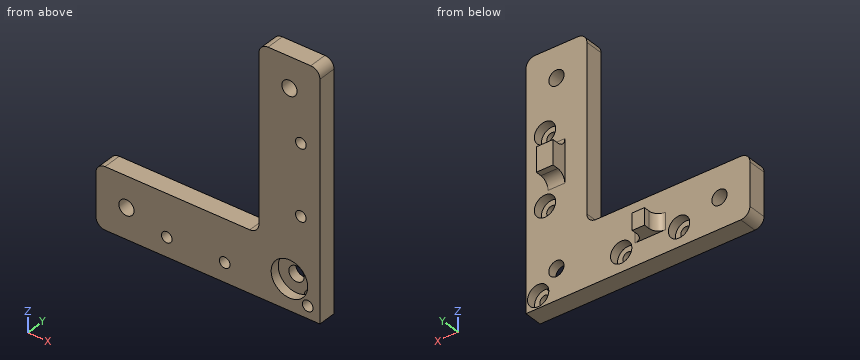
Autodesk Inventor part; units mm, degrees
ref_plane "YZ Plane" through (0, 0, 0) normal (1, 0, 0) x (0, 1, 0)
ref_plane "XZ Plane" through (0, 0, 0) normal (0, 1, 0) x (-1, 0, 0)
ref_plane "XY Plane" through (0, 0, 0) normal (0, 0, 1) x (1, 0, 0)
sketch "Эскиз1" plane through (0, 0, 0) normal (0, 1, 0) x (-1, 0, 0)
  line L0 (0, 0) -> (0, 80)
  line L1 (0, 80) -> (20, 80)
  line L2 (20, 80) -> (20, 20)
  line L3 (20, 20) -> (73.5, 20)
  line L4 (73.5, 20) -> (73.5, 0)
  line L5 (73.5, 0) -> (0, 0)
  dimension "d0" = 80
  dimension "d1" = 20
  dimension "d2" = 60
  dimension "d3" = 53.5
extrude "Выдавливание1" add sketch "Эскиз1" along normal blind 6
fillet "Сопряжение1" radius 3 5 edges at (-73.5, 3, 20) (-73.5, 3, 0) (-20, 3, 80) (0, 3, 80) (-20, 3, 20)
sketch "Эскиз2" plane through (0, 6, 0) normal (0, 1, 0) x (1, 0, 0)
  circle A0 centre (-6.25, -31.25) radius 1.75
  circle A1 centre (-4, -4) radius 1.75
  circle A2 centre (-31.25, -6.25) radius 1.75
  circle A3 centre (-50.25, -6.25) radius 1.75
  circle A4 centre (-6.25, -54.25) radius 1.75
  circle A5 centre (-6.25, -54.25) radius 3.5
  circle A6 centre (-6.25, -31.25) radius 3.5
  circle A7 centre (-4, -4) radius 3.5
  circle A8 centre (-31.25, -6.25) radius 3.5
  circle A9 centre (-50.25, -6.25) radius 3.5
  dimension "d7" = 7
  dimension "d8" = 7
  dimension "d9" = 7
  dimension "d10" = 7
  dimension "d11" = 7
extrude "Выдавливание2" cut sketch "Эскиз2" against normal through all contours A0 | A1 | A2 | A3 | A4
extrude "Выдавливание3" cut sketch "Эскиз2" against normal blind 3 contours A0 | A1 | A2 | A3 | A4 | A5 | A6 | A7 | A8 | A9
sketch "Эскиз3" plane through (0, 6, 0) normal (0, 1, 0) x (1, 0, 0)
  line L0 (-20, -85.5935) -> (0, -85.5935)
  line L1 (-7.25, -46.75) -> (-12.75, -46.75)
  line L2 (-12.75, -46.75) -> (-12.75, -38.75)
  line L3 (-12.75, -38.75) -> (-7.25, -38.75)
  line L4 (-7.25, -38.75) -> (-7.25, -46.75)
  line L5 (-7.25, -46.75) -> (-12.75, -38.75) construction
  line L6 (-12.75, -46.75) -> (-7.25, -38.75) construction
  line L7 (0, 0) -> (13.4319, 0) construction
  line L8 (-42.75, -12.75) -> (-38.75, -12.75)
  line L9 (-38.75, -12.75) -> (-38.75, -7.25)
  line L10 (-38.75, -7.25) -> (-42.75, -7.25)
  line L11 (-42.75, -7.25) -> (-42.75, -12.75)
  point P0 (-10, -42.75)
extrude "Выдавливание4" add sketch "Эскиз3" along normal blind 5
sketch "Эскиз4" plane through (0, 6, 0) normal (0, 1, 0) x (1, 0, 0)
  line L0 (-27.1384, -80) -> (-27.1384, -70)
  line L1 (-80, 9.988) -> (-53.75, 9.988)
  circle A0 centre (-10, -70) radius 2.5
  line L2 (-73.5, -29.8806) -> (-63.5, -29.8806)
  circle A1 centre (-63.5, -10) radius 2.5
  point P0 (0, 0)
  dimension "d26" = 10
  dimension "d27" = 5
  dimension "d28" = 10
  dimension "d29" = 5
extrude "Выдавливание5" cut sketch "Эскиз4" against normal through all
sketch "Эскиз5" plane through (0, 0, 0) normal (0, -1, 0) x (1, 0, 0)
  line L0 (0, 77) -> (0, 0)
  line L1 (0, 0) -> (-10, 0)
  line L2 (-10, 0) -> (-10, 10)
  line L3 (-10, 10) -> (0, 10)
  line L4 (0, 10) -> (0, 0)
  circle A0 centre (-10, 10) radius 2.5
  circle A1 centre (-10, 10) radius 6
  dimension "d32" = 10
  dimension "d33" = 10
  dimension "d34" = 5
  dimension "d35" = 12
extrude "Выдавливание6" cut sketch "Эскиз5" against normal through all contours A0 L2 L3 | L3 L2 A0
extrude "Выдавливание7" cut sketch "Эскиз5" against normal blind 3 contours A1 L2 A0 L3 | L3 A0 L2 A1 | A0 L2 L3 | L3 L2 A0
fillet "Сопряжение2" radius 3 4 edges at (-42.75, 6, 10) (-38.75, 6, 10) (-10, 6, 38.75) (-10, 6, 46.75)
properties part number "perehodnik"
Here's how the part is built. I have some questions about the finished solid (model axes, mm). Give positions to 0.01 mm unless a question says otherwise; leave off trailing zeros. Write each loop counter-clockwise with the first axis right and the second up, starting at its lowest first coordinate (ties: lowest second). Pieces come first, ordered by that corner, then holes. Notation, with made-up numbers: (11.5, -31.75) -> (18.5, -31.75) arc R20 ccw to (18.5, 6.25) -> close; hole circle Ø7 at (48.25, 56.5). An arc over 180 degrees is marked (long way). Write each question's results on one line, items separated by ' | '.
Item 1: Suppose I cut it at C-C on x = -63.5. Write out the boundary of the cut face in (y, z), plus the area to 3 significant figures.
Output:
outline: (0, 0) -> (6, 0) -> (6, 7.5) -> (0, 7.5) -> close; (0, 12.5) -> (6, 12.5) -> (6, 20) -> (0, 20) -> close | area: 90.0 mm^2
Item 2: Suppose I cut it at B-B on y = 4. Give the number of separate pieces and of enclosed holes in the cut face, plus the area to 3 significant figures.
Output:
separate pieces: 1 | enclosed holes: 8 | area: 2,410 mm^2
Item 3: If I drill on L1, parallel to X at y = 4.75, z = 31.25; L2, parallel to Z at x = -10, y = 0.9; L3, parallel to X at y = 2.05, z = 31.25, over which ranges is the centre line in solid material (lowest first)?
Output:
L1: x = -20 to -9.75, -2.75 to 0 | L2: z = 0 to 4, 16 to 67.5, 72.5 to 80 | L3: x = -20 to -8, -4.5 to 0
Item 4: Suppose I cut it at D-D on z = 31.25. Write out the boundary of the cut face in (x, y).
Output:
outline: (-20, 0) -> (-8, 0) -> (-8, 3) -> (-9.75, 3) -> (-9.75, 6) -> (-20, 6) -> close; (-4.5, 0) -> (0, 0) -> (0, 6) -> (-2.75, 6) -> (-2.75, 3) -> (-4.5, 3) -> close
Item 5: Suppose I cut it at A-A on z = 70. Write out the boundary of the cut face in (x, y).
Output:
outline: (-20, 0) -> (-12.5, 0) -> (-12.5, 6) -> (-20, 6) -> close; (-7.5, 0) -> (0, 0) -> (0, 6) -> (-7.5, 6) -> close
Item 6: For pin 1 Ø5.5 at (x, y) = (-43, 8.5) entering from +Z; pin 2 Ø3.5 at (x, z) = (-4, 3.5) entering from +Y; pin 3 Ø3.5 at (x, z) = (-13, 12) entering from -Y; pin 4 Ø4 at (x, z) = (-10, 70) entering from -Y, each with a flat end and sliding along its axis, tell me the tip position at first contact or that it passes through.
Output:
pin 1: stops at z = 20 | pin 2: stops at y = 3 | pin 3: stops at y = 3 | pin 4: passes through
